```python
from build123d import *

# Parameters (mm, degrees)
F0_W     = 255
F0_H     = 250
F1_DEPTH = 117
F2_T     = -3
F3_W     = 255
F3_H     = 250
F4_DEPTH = 3
F5_R     = 20
F6_DEPTH = 25
F7_R     = 15
F8_DEPTH = 20
F9_R     = 15


with BuildPart() as f1:
    # F0 (on Top) → F1 (new body)
    with BuildSketch(Plane.XY):
        Rectangle(F0_W, F0_H)
    extrude(amount=F1_DEPTH)

    # F2
    f2_openings = [f1.faces().sort_by_distance(p)[0] for p in [
        (0, 0, 117),
    ]]
    offset(amount=F2_T, openings=f2_openings)

    # F3 (on face) → F4 (join)
    with BuildSketch(Plane.XY.offset(117)):
        Rectangle(F3_W, F3_H)
    extrude(amount=F4_DEPTH)

    # F5 (on face) → F6 (cut)
    with BuildSketch(Plane.XZ.offset(125)):
        with Locations((0, 60)):
            Circle(F5_R)
    extrude(amount=-F6_DEPTH, mode=Mode.SUBTRACT)

    # F7 (on face) → F8 (join)
    with BuildSketch(Plane.XY.offset(120)):
        with Locations((-80, 40)):
            Circle(F7_R)
        with Locations((0, 40)):
            Circle(F7_R)
        with Locations((80, 40)):
            Circle(F7_R)
        with Locations((-80, -45)):
            Circle(F7_R)
        with Locations((0, -45)):
            Circle(F7_R)
        with Locations((80, -45)):
            Circle(F7_R)
    extrude(amount=F8_DEPTH)

    # F9
    f9_edges = [f1.edges().sort_by_distance(p)[0] for p in [
        (-15, 40, 140),
        (-95, 40, 140),
        (65, 40, 140),
        (65, -45, 140),
        (-15, -45, 140),
        (-95, -45, 140),
    ]]
    fillet(f9_edges, radius=F9_R)


solid = f1.part
```
CAD build for the part. Positions are in the model's coordinates, mm. A direction names the side the tool comes from. Give positions to 0.01 mm unless a question says otherwise; leave off trailing zeros. Order: outer loops, then holes, each group sorted by start corner. A loop starts at its lowest first (then second) coordinate and runs counter-clockwise, first axis right, second up.
(1) Flat gauge pins, fed straight in: pin 1 (2 mm diameter, centred on x = 75.5, y = 40, fed in from +Z); pin 2 (6 mm diameter, centred on x = 21, y = 66.5, fed in from +Z). Where does each tip first touch, or does it go through?
(2) Saw through at A-A, the plane x = -109.5. Give the cut face in (y, z).
(3) Saw through at B-B, the plane y = 70. Give the cut face in (x, z), then the cut area to 3 significant figures.
(4) Tool access for faces 1 (the cylindrical face through (-71.94, 52.65, 122.46)), 2 (the flat face through (-2, 125, 59)), 3 (the flat face through (-127.5, -2, 59)), 4 (the flat face through (124.5, -2, 59)), 5 (the cylindrical face through (-4.336, -123.521, 40.476)): list every direction of +Z, -Z, +X, -X, +Y, -Y with a clear straight run to the whole face (end or side of a thin tool).
(5) Mould opens along X. For faces 6 (the flat face through (127.5, -2, 59)), 7 (the flat face through (-2, 2, 117)), 8 (the flat face through (-2, -125, 32)) say: released by +X, released by -X, zero draft, split by the parting line, or undercut.
(6) Saw through at C-C, the plane z = 60. Give the cut face in (x, y).
(7) Drill centre lines: L1, parallel to Z at x = -80, y = -81; L2, parallel to Z at x = 0, y = -123.2; L3, parallel to Y at x = -33, z = 33. Where is each one in solid material? Low to high.
(8) Saw through at D-D, the plane x = 0. Give the cut face in (y, z).
Results found:
1. pin 1: stops at z = 139.59
1. pin 2: stops at z = 120
2. outline: (-125, 0) - (125, 0) - (125, 120) - (-125, 120) - close; hole (-122, 3) - (122, 3) - (122, 117) - (-122, 117) - close
3. outline: (-127.5, 0) - (127.5, 0) - (127.5, 120) - (-127.5, 120) - close; hole (-124.5, 3) - (124.5, 3) - (124.5, 117) - (-124.5, 117) - close
3. area: 2,210 mm2
4. face 1: +Z
4. face 2: +Z, -Z, +X, -X, +Y
4. face 3: +Z, -Z, -X, +Y, -Y
4. face 4: none
4. face 5: -Y
5. face 6: released by +X
5. face 7: undercut
5. face 8: zero draft
6. outline: (-127.5, -125) - (-20, -125) - (-20, -122) - (-124.5, -122) - (-124.5, 122) - (124.5, 122) - (124.5, -122) - (20, -122) - (20, -125) - (127.5, -125) - (127.5, 125) - (-127.5, 125) - close
7. L1: z = 0 to 3, 117 to 120
7. L2: z = 0 to 40, 80 to 120
7. L3: y = -125 to -122, 122 to 125
8. outline: (-125, 0) - (125, 0) - (125, 120) - (55, 120) - (55, 125) arc R15 ccw to (25, 125) - (25, 120) - (-30, 120) - (-30, 125) arc R15 ccw to (-60, 125) - (-60, 120) - (-125, 120) - (-125, 80) - (-122, 80) - (-122, 117) - (122, 117) - (122, 3) - (-122, 3) - (-122, 40) - (-125, 40) - close
